from build123d import *

# Parameters (mm, degrees)
TALADRO_DE_MARGEN_PARA_M102_D     = 12
TALADRO_DE_MARGEN_PARA_M102_DEPTH = 55.394836286
TALADRO_DE_MARGEN_PARA_M102_TIP   = 3.605163714


with BuildPart() as part:
    # Croquis1 → Revolución1 (revolve)
    with BuildSketch(Plane.XY):
        Polygon((100, 0), (100, 12), (99.5, 12.5), (83.5, 12.5), (80.481641108, 47), (77.481641108, 50), (-77.481641108, 50), (-80.481641108, 47), (-83.5, 12.5), (-99.5, 12.5), (-100, 12), (-100, 0), align=None)
    revolve(axis=Axis((112.244897959, 0, 0), (-1, 0, 0)))

    # Croquis8 → Taladro de margen para M101 (revolve, cut)
    with BuildSketch(Plane(origin=(-100, 0, 0), x_dir=(0, 0, 1), z_dir=(0, 1, 0))):
        Polygon((0, 0), (0, 59), (6, 55.394836286), (6, 0), align=None)
    revolve(axis=Axis((-106.35, 0, 0), (1, 0, 0)), mode=Mode.SUBTRACT)

    # Taladro de margen para M102
    with Locations(Plane(origin=(100, 0, 0), x_dir=(0, 0, 1), z_dir=(1, 0, 0))):
        with Locations((0, 0)):
            Hole(TALADRO_DE_MARGEN_PARA_M102_D / 2, depth=TALADRO_DE_MARGEN_PARA_M102_DEPTH)
            with Locations((0, 0, -(TALADRO_DE_MARGEN_PARA_M102_DEPTH + TALADRO_DE_MARGEN_PARA_M102_TIP / 2))):  # 118° drill point
                Cone(0, TALADRO_DE_MARGEN_PARA_M102_D / 2, TALADRO_DE_MARGEN_PARA_M102_TIP, mode=Mode.SUBTRACT)


solid = part.part
The listing builds one solid part. Answer for the finished solid, in the listing's coordinates (mm). A direction names the side the tool comes from. Give positions to 0.01 mm unless a question says otherwise; leave off trailing zeros. Write each loop counter-clockwise with the first axis right and the second up, starting at its lowest first coordinate (ties: lowest second). Pieces come first, ordered by that corner, then holes. Notation, with made-up numbers: (11.5, -12) -> (20.5, -12) arc R30 cw to (20.5, 10) -> close; hole circle Ø6 at (85.25, 7.25). An arc over 180 degrees is marked (long way). Use a Markdown table: item, result.
(1) Flat-ended cylindrical pins translate along their axes: P1, Ø11, axis at y = 0, z = 0, coming from the +X side; P2, Ø3, axis at x = 16.5, z = 13.5, coming from the -Y side; P3, Ø5, axis at y = -32, z = 35.5, coming from the -X side. Find the tip coordinate at first contact, or state that the pin passes through.
Return value:
| item | result |
|---|---|
| P1 | x = 44.3 |
| P2 | y = -48.54 |
| P3 | x = -80.63 |
(2) Determine the mould class of faces 4 (the conical face through (80.29, -10.23, 46.07)), 5 (the flat face through (100, 6, 2)), 6 (the cylindrical face through (72, 0, 6)) for opening direction Z: released by +Z, released by -Z, zero draft, split by the parting line, or undercut.
Return value:
| item | result |
|---|---|
| face 4 | split by the parting line |
| face 5 | zero draft |
| face 6 | undercut |
(3) Section A-A, the plane x = -8 is taken. Determine the outline of the cut face in (y, z).
Return value:
| item | result |
|---|---|
| outline | circle Ø100 at (0, 0) |
(4) Find the intervals of material crossed by probe 1 along Y at (x, z) = (-67, 0); probe 2 along Z at (x, y) = (-15, 1.5), in increasing order. Write a range as from..to.
Return value:
| item | result |
|---|---|
| probe 1 | -50..-6, 6..50 |
| probe 2 | -49.98..49.98 |
(5) For faces 1 (the flat face through (-100, -6, 2)), 2 (the cylindrical face through (91.388, 11.923, -3.755)), 3 (the cylindrical face through (-73, 0, -6)), determine the directions among +Z, -Z, +X, -X, +Y, -Y from which every point of the face is accessible in a straight line to the end or side of a thin tool.
Return value:
| item | result |
|---|---|
| face 1 | +Z, -Z, -X, +Y, -Y |
| face 2 | +X |
| face 3 | -X |
